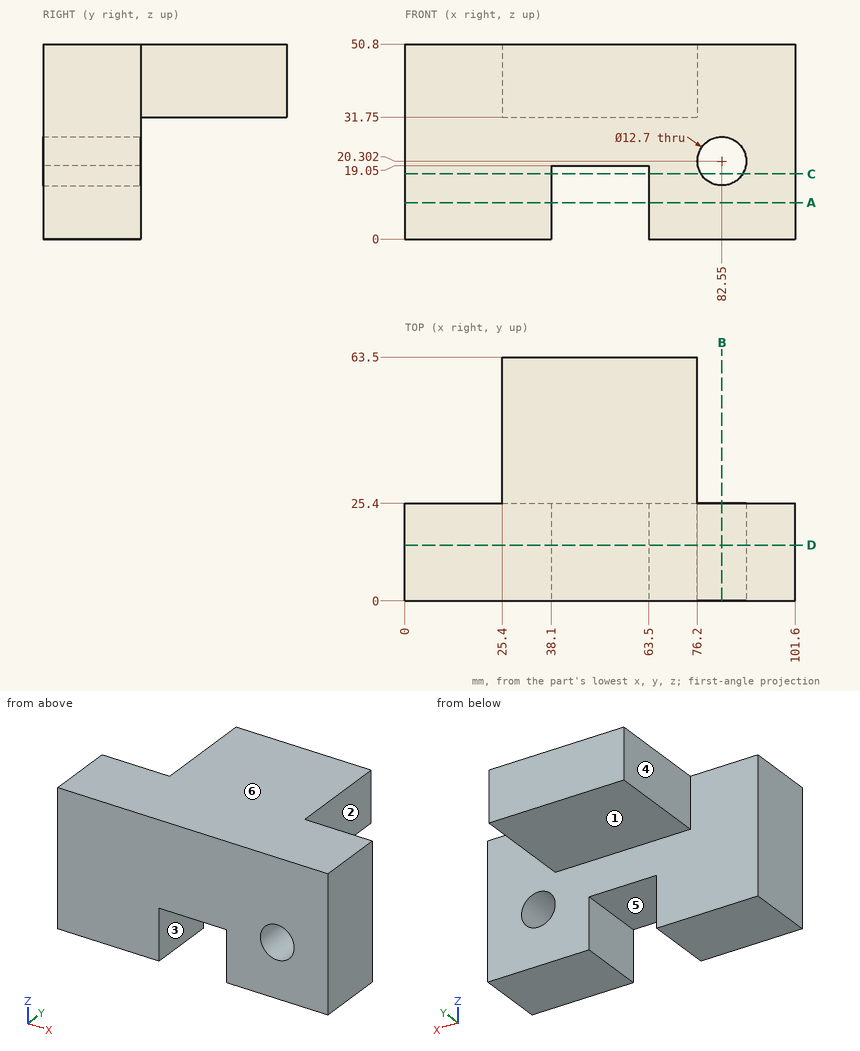
Source: three-view drawing plus pictorial views. Frame: mm from the lowest corner of the part. A direction names the side the tool comes from. Round coordinates to 2 decimals unless told otherwise and drop trailing zeros. Loops run counter-clockwise (first coordinate to the right, second up) from the corner with the lowest first, then second, coordinate; pieces in that order, holes last. Notation, with made-up numbers: (-3.5, 74) -> (45.5, 74) arc R26 ccw to (45.5, 107) -> close; hole circle Ø11 at (18, 33). An arc over 180 degrees is marked (long way). Use one line per item in the form item = value.
Item 1: Access query for the marked faces 4, 5 and 6. Directions: +Z, -Z, +X, -X, +Y, -Y. A direction counts if a zero-diameter tool reaches every point of the face in a straight line with its end or side. Return the directions, or none.
Evaluation:
face_4 = +Z, -Z, -X, +Y
face_5 = -Z, +Y, -Y
face_6 = +Z, +X, -X, +Y, -Y
Item 2: Cut plane C-C on z = 17. Output: boundary loops of the cut face in (x, y) (1 decimal), then the cut area to 3 significant figures.
Evaluation:
outline = (0, 0) -> (38.1, 0) -> (38.1, 25.4) -> (0, 25.4) -> close; (63.5, 0) -> (77.1, 0) -> (77.1, 25.4) -> (63.5, 25.4) -> close; (88, 0) -> (101.6, 0) -> (101.6, 25.4) -> (88, 25.4) -> close
area = 1,660 mm2
Item 3: Contact query for flat-ended pins moving along their axis: pin 1 Ø7.5 at (x, z) = (82.55, 20.3) entering from +Y; pin 2 Ø12.5 at (x, y) = (51.5, 12.5) entering from -Z; pin 3 Ø5.5 at (y, z) = (51.5, 38.5) entering from +X; pin 4 Ø21 at (y, z) = (53, 42.5) entering from -X. Output: stop coordinate, or through.
Evaluation:
pin_1 = through
pin_2 = 19.05
pin_3 = 76.2
pin_4 = 25.4
Item 4: Cut plane A-A on z = 9.5. Output: boundary loops of the cut face in (x, y), then the cut area to 3 significant figures.
Evaluation:
outline = (0, 0) -> (38.1, 0) -> (38.1, 25.4) -> (0, 25.4) -> close; (63.5, 0) -> (101.6, 0) -> (101.6, 25.4) -> (63.5, 25.4) -> close
area = 1,940 mm2
Item 5: Material intervals for probe 1 along Z at (x, y) = (82, 18) (1 decimal); probe 2 along Z at (x, y) = (82.55, 9.75); probe 3 along Y at (x, z) = (30, 17.5), sorted ascending.
Evaluation:
probe_1 = 0 to 14, 26.6 to 50.8
probe_2 = 0 to 13.95, 26.65 to 50.8
probe_3 = 0 to 25.4
Item 6: Cut plane D-D on y = 14.5. Output: boundary loops of the cut face in (x, z), then the cut area to 3 significant figures.
Evaluation:
outline = (0, 0) -> (38.1, 0) -> (38.1, 19.05) -> (63.5, 19.05) -> (63.5, 0) -> (101.6, 0) -> (101.6, 50.8) -> (0, 50.8) -> close; hole circle Ø12.7 at (82.55, 20.3)
area = 4,550 mm2
Item 7: Draft query along X for the marked faces 1, 2 and 3. Return one class per face: released by +X, released by -X, zero draft, split by the parting line, or undercut.
Evaluation:
face_1 = zero draft
face_2 = released by +X
face_3 = undercut
Item 8: Cut plane B-B on x = 82.55. Output: boundary loops of the cut face in (y, z).
Evaluation:
outline = (0, 0) -> (25.4, 0) -> (25.4, 13.95) -> (0, 13.95) -> close; (0, 26.65) -> (25.4, 26.65) -> (25.4, 50.8) -> (0, 50.8) -> close
